Could you check a few things on this model? Use its own coordinates, in mm. Face numbers are marked on the shaded views. A direction names the side the tool comes from. Coordinates: 2 decimals unless noted, no trailing zeros. Write each loop counter-clockwise with the first axis right and the second up, starting at its lowest first coordinate (ties: lowest second). Pieces come first, ordered by that corner, then holes.
```python
from build123d import *

# Parameters (mm, degrees)
BOSS_EXTRUDE1_DEPTH = 2.5
SKETCH2_R           = 1.25
CUT_EXTRUDE1_DEPTH  = 7.931238628
SKETCH3_R           = 1.75
CUT_EXTRUDE2_DEPTH  = 8
FILLET1_R           = 2


with BuildPart() as part:
    # Sketch1 → Boss-Extrude1 (new body, symmetric)
    with BuildSketch(Plane.XY):
        Polygon((16, -1.5), (16, -3.5), (0, -3.5), (-1.835919027, 0.43714106), (-7.27376575, -2.098568511), (-7.696384011, -1.192260724), (-2.258537289, 1.343448847), (-2.892464682, 2.702910527), (-8.330311404, 0.167200957), (-8.752929666, 1.073508744), (-0.633927393, 4.859461681), (0, 3.5), (16, 3.5), (16, 1.5), (4, 1.5), (4, -1.5), align=None)
    extrude(amount=BOSS_EXTRUDE1_DEPTH, both=True)

    # Sketch2 → Cut-Extrude1 (cut, through all)
    with BuildSketch(Plane(origin=(-0.495341252, 1.062262743, 0), x_dir=(0.906307787, 0.422618262, 0), z_dir=(0.422618262, -0.906307787, 0))):
        with Locations((-4.979163916, 0)):
            Circle(SKETCH2_R)
    extrude(amount=-CUT_EXTRUDE1_DEPTH, mode=Mode.SUBTRACT)

    # Sketch3 → Cut-Extrude2 (cut, through all)
    with BuildSketch(Plane(origin=(0, 3.5, 0), x_dir=(1, 0, 0), z_dir=(0, 1, 0))):
        with Locations((12, 0)):
            Circle(SKETCH3_R)
    extrude(amount=-CUT_EXTRUDE2_DEPTH, mode=Mode.SUBTRACT)

    # Fillet1
    fillet1_edges = [part.edges().sort_by_distance(p)[0] for p in [
        (-7.485074881, -1.645414617, -2.5),
        (-8.541620535, 0.62035485, -2.5),
        (16, 2.5, -2.5),
        (16, -2.5, -2.5),
        (16, 2.5, 2.5),
        (-8.541620535, 0.62035485, 2.5),
        (16, -2.5, 2.5),
        (-7.485074881, -1.645414617, 2.5),
    ]]
    fillet(fillet1_edges, radius=FILLET1_R)


solid = part.part
```
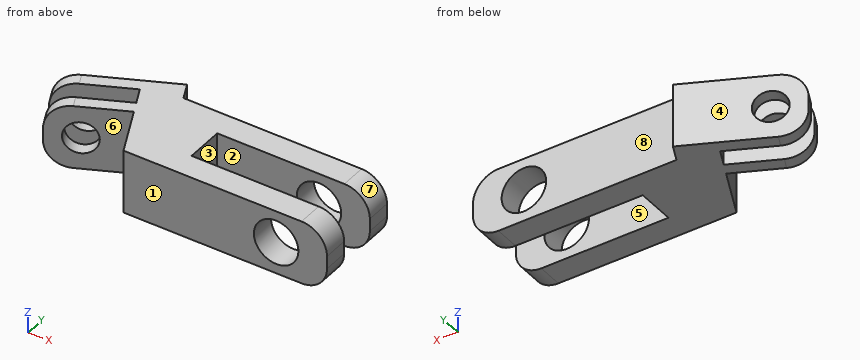
Item 1: Which directions (+Z, -Z, +X, -X, +Y, -Y) give clear straight access to the entire face, cutting with the end or side of a thin tool? Please do the marked faces 5, 6, 7 and 8.
Item 2: If we mould it in two halves opening along Y, with no side actions, what happens to the marked faces 1, 2, 3 and 4? For each: released by +Y, released by -Y, zero draft, split by the parting line, or undercut.
Item 3: I want a section at A-A, the plane x = 12. List the corners of the cut face in (y, z) for me.
Item 4: I want a section at C-C, the plane x = -3.5. List the corners of the cut face in (y, z) for me, then the cut area to 3 significant figures.
Item 5: Will these pins go through, and if not, where does the flat tip stop? pin 1 Ø1.5 at (y, z) = (0.5, 0) entering from +X; pin 2 Ø1.5 at (y, z) = (-1, -1.5) entering from +X.
Item 6: If I drill on line 1 along Y through (x, z) = (13.25, -1.9); line 2 along Z through (x, y) = (12, 2.35); line 3 along X through (y, z) = (2.1, 0), over which ranges is the centre line in solid material (lowest first)?
Item 7: I want a section at B-B, the plane z = -1. Count the separate pieces of the cut face and the enclosed holes in it, then the cut area to 3 significant figures.
Item 8: I want a section at D-D, the plane y = 3.25. List the corners of the cut face in (x, z) for me, then the cut area to 3 significant figures.
Taken from the geometry:
1. face 5: +Z, -Z, +X
1. face 6: +Z, -Z, -Y
1. face 7: +Z, +X, +Y, -Y
1. face 8: +Z, -Z, +X, +Y
2. face 1: released by -Y
2. face 2: undercut
2. face 3: undercut
2. face 4: released by +Y
3. outline: (-3.5, -2.5) - (-1.5, -2.5) - (-1.5, -1.75) - (-3.5, -1.75) - close; (-3.5, 1.75) - (-1.5, 1.75) - (-1.5, 2.5) - (-3.5, 2.5) - close; (1.5, -2.5) - (3.5, -2.5) - (3.5, -1.75) - (1.5, -1.75) - close; (1.5, 1.75) - (3.5, 1.75) - (3.5, 2.5) - (1.5, 2.5) - close
4. outline: (-0.34, -2.5) - (0.76, -2.5) - (0.76, 2.5) - (-0.34, 2.5) - close; (2.42, -2.5) - (3.52, -2.5) - (3.52, 2.5) - (2.42, 2.5) - close
4. area: 11.0 mm2
5. pin 1: stops at x = 4
5. pin 2: stops at x = 15.95
6. line 1: y = -3.5 to -1.5, 1.5 to 3.5
6. line 2: z = -2.5 to -1.75, 1.75 to 2.5
6. line 3: x = -5.09 to -4.19, -2.61 to 10.25, 13.75 to 16
7. separate pieces: 5
7. enclosed holes: 0
7. area: 87.0 mm2
8. outline: (-4.09, -2.5) - (14, -2.5) arc R2 ccw to (16, -0.5) - (16, 0.5) arc R2 ccw to (14, 2.5) - (-4.09, 2.5) - close; hole circle Ø3.5 at (12, 0)
8. area: 89.1 mm2
